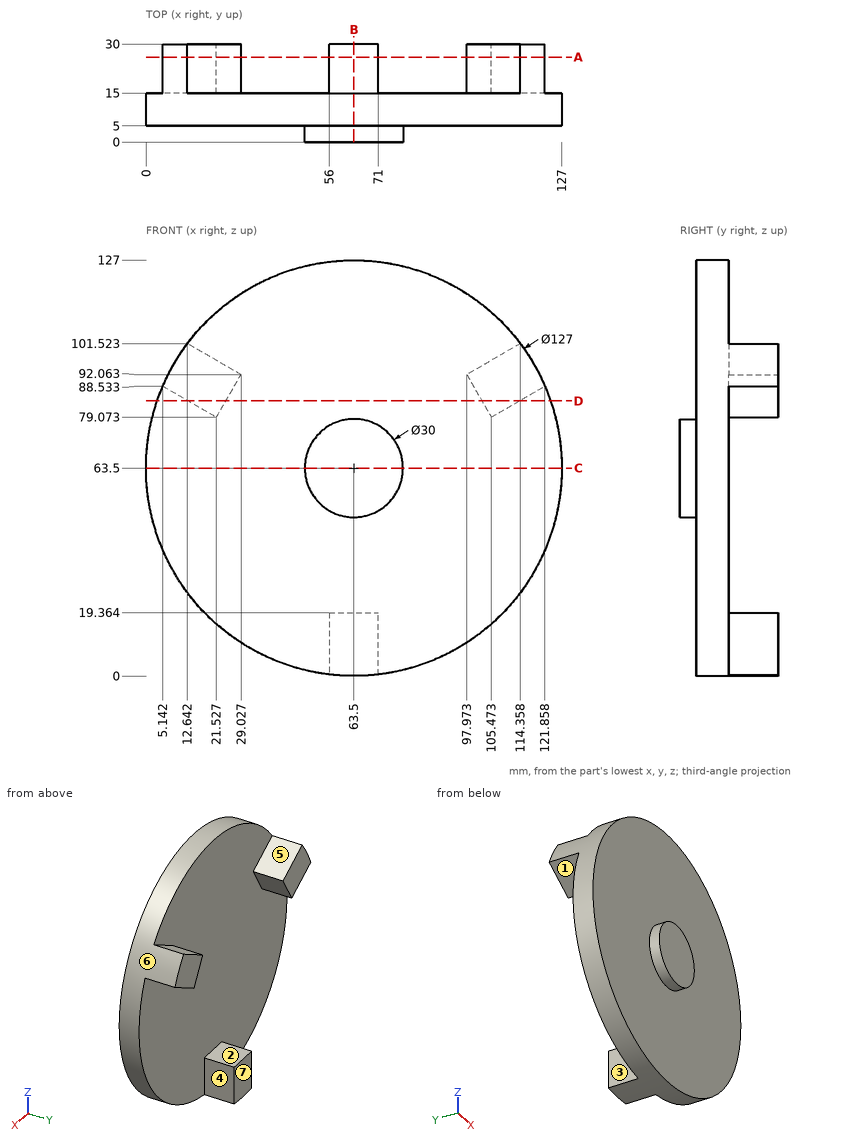
Could you check a few things on this drawing? It's one solid part, dimensions in mm from its lowest x, y, z. A direction names the side the tool comes from. Give positions to 0.01 mm unless a question says otherwise; leave off trailing zeros. Order: outer loops, then holes, each group sorted by start corner. A loop starts at its lowest first (then second) coordinate and runs counter-clockwise, first axis right, second up.
1. Suppose I cut it at D-D (z = 84). Write out the boundary of the cut face in (x, y).
Answers below:
outline: (3.4, 5) - (123.6, 5) - (123.6, 15) - (114.01, 15) - (114.01, 30) - (102.63, 30) - (102.63, 15) - (24.37, 15) - (24.37, 30) - (12.99, 30) - (12.99, 15) - (3.4, 15) - close
2. I need wall thicknesses on L1, parallel to Y at x = 69, z = 34.5; L2, parallel to Y at x = 66, z = 9; L3, parallel to Z at x = 62.5, y = 1.75. Which ranges of each line are inside material? Lowest first, please.
Answers below:
L1: y = 5 to 15
L2: y = 5 to 30
L3: z = 48.53 to 78.47
3. Which directions (+Z, -Z, +X, -X, +Y, -Y) give clear straight access to the entire face, cutting with the end or side of a thin tool? Please do the marked faces 1, 2, 3 and 4.
Answers below:
face 1: -Z, -X, +Y
face 2: +Z, +X, -X, +Y
face 3: +Z, -Z, -X, +Y
face 4: +Z, -Z, +X, +Y
4. For pin 1 (4 mm diameter, centred on y = 6.5, z = 17.5, fed in from -X) (1 decimal); pin 2 (4.5 mm diameter, centred on x = 64.5, y = 20.5, fed in from +Z); pin 3 (6 mm diameter, centred on x = 68.5, y = 10.5, fed in from +Z), each with a flat end and sliding along its axis, tell me the tip position at first contact or that it passes through.
Answers below:
pin 1: stops at x = 17.7
pin 2: stops at z = 19.36
pin 3: stops at z = 126.97
5. Suppose I cut it at B-B (x = 63.5). Write out the boundary of the cut face in (y, z), plus the area to 3 significant figures.
Answers below:
outline: (0, 48.5) - (5, 48.5) - (5, 0) - (30, 0) - (30, 19.36) - (15, 19.36) - (15, 127) - (5, 127) - (5, 78.5) - (0, 78.5) - close
area: 1,710 mm2
6. Suppose I cut it at C-C (z = 63.5). Write out the boundary of the cut face in (x, y).
Answers below:
outline: (0, 5) - (48.5, 5) - (48.5, 0) - (78.5, 0) - (78.5, 5) - (127, 5) - (127, 15) - (0, 15) - close
7. Thinking about a two-plate mould opening in X: for the marked faces 5, 6 and 7, which applies, +X half, -X half, draft (parallel to the pull), parting line (faces both ways), or undercut?
Answers below:
face 5: undercut
face 6: parting line
face 7: draft
8. Suppose I cut it at A-A (y = 26). Write out the boundary of the cut face in (x, z) (1 decimal).
Answers below:
outline: (5.1, 88.5) - (21.5, 79.1) - (29, 92.1) - (12.6, 101.5) arc R63.5 ccw to start; (56, 0.4) arc R63.5 ccw to (71, 0.4) - (71, 19.4) - (56, 19.4) - close; (98, 92.1) - (105.5, 79.1) - (121.9, 88.5) arc R63.5 ccw to (114.4, 101.5) - close
